```python
from build123d import *

# Parameters (mm, degrees)
BOSS_EXTRUDE1_DEPTH     = 25.5
SKETCH2_R               = 22.5
BOSS_EXTRUDE2_DEPTH     = 100
SKETCH3_W               = 30
SKETCH3_H               = 32
BOSS_EXTRUDE3_DEPTH     = 164.7
SKETCH4_W               = 19
SKETCH4_H               = 20
BOSS_EXTRUDE4_DEPTH     = 20
SKETCH5_R               = 4.05
CUT_EXTRUDE1_DEPTH      = 202.549720913
SKETCH6_R               = 10
BOSS_EXTRUDE5_DEPTH     = 25
SKETCH7_W               = 33
SKETCH7_H               = 35
BOSS_EXTRUDE6_DEPTH     = 13
CUT_EXTRUDE2_DEPTH      = 225.141785484
CUT_EXTRUDE2_DEPTH_BACK = 225.141785484
SKETCH8_R               = 4.05
FILLET1_R               = 2
CUT_EXTRUDE3_START      = -100
SKETCH9_R               = 10
CUT_EXTRUDE3_DEPTH      = 100


with BuildPart() as part:
    # Sketch1 → Boss-Extrude1 (new body)
    with BuildSketch(Plane.XY):
        with BuildLine():
            Line((-22, -4.716990566), (-22, -58.5))
            Line((-22, -58.5), (22, -58.5))
            Line((22, -58.5), (22, -4.716990566))
            ThreePointArc((22, -4.716990566), (0, 22.5), (-22, -4.716990566))
        make_face()
    extrude(amount=BOSS_EXTRUDE1_DEPTH)

    # Sketch2 → Boss-Extrude2 (add)
    with BuildSketch(Plane.XY.offset(25.5)):
        with Locations(Location((0, 0, 0), (0, 0, 192.101492032))):
            Circle(SKETCH2_R)
    extrude(amount=BOSS_EXTRUDE2_DEPTH)

    # Sketch3 → Boss-Extrude3 (add)
    with BuildSketch(Plane.XY.offset(25.5)):
        with Locations((0, -41)):
            Rectangle(SKETCH3_W, SKETCH3_H)
    extrude(amount=BOSS_EXTRUDE3_DEPTH)

    # Sketch4 → Boss-Extrude4 (add)
    with BuildSketch(Plane(origin=(0, 0, 0), x_dir=(-1, 0, 0), z_dir=(0, 0, -1))):
        with Locations((0, -37.7)):
            Rectangle(SKETCH4_W, SKETCH4_H)
    extrude(amount=BOSS_EXTRUDE4_DEPTH)

    # Sketch5 → Cut-Extrude1 (cut, through all)
    with BuildSketch(Plane(origin=(9.5, 0, 0), x_dir=(0, 0, -1), z_dir=(1, 0, 0))):
        with Locations((11, -37.7)):
            Circle(SKETCH5_R)
    extrude(amount=-CUT_EXTRUDE1_DEPTH, mode=Mode.SUBTRACT)

    # Sketch6 → Boss-Extrude5 (add)
    with BuildSketch(Plane.XY.offset(190.2)):
        with Locations((0, -37.7)):
            Circle(SKETCH6_R)
    extrude(amount=BOSS_EXTRUDE5_DEPTH)

    # Sketch7 → Boss-Extrude6 (add)
    with BuildSketch(Plane.XY.offset(190.2)):
        with Locations((0, -41)):
            Rectangle(SKETCH7_W, SKETCH7_H)
    extrude(amount=-BOSS_EXTRUDE6_DEPTH)

    # Sketch8 → Cut-Extrude2 (cut, two sides: drawn at the far end of the back side and taken through both)
    with BuildSketch(Plane(origin=(0, 0, 0), x_dir=(0, 0, -1), z_dir=(1, 0, 0)).offset(-CUT_EXTRUDE2_DEPTH_BACK)):
        with Locations(Location((-205.2, -37.7, 0), (0, 0, 179.999999993))):
            Circle(SKETCH8_R)
    extrude(amount=CUT_EXTRUDE2_DEPTH + CUT_EXTRUDE2_DEPTH_BACK, mode=Mode.SUBTRACT)

    # Fillet1
    fillet1_edges = [part.edges().sort_by_distance(p)[0] for p in [
        (15, -57, 101.35),
        (-15, -57, 101.35),
        (-15, -25, 101.35),
        (15, -25, 101.35),
    ]]
    fillet(fillet1_edges, radius=FILLET1_R)

    # Sketch9 → Cut-Extrude3 (cut)
    with BuildSketch(Plane.XY.offset(215.2).offset(CUT_EXTRUDE3_START)):
        with Locations((0, -37.7)):
            Circle(SKETCH9_R)
    extrude(amount=CUT_EXTRUDE3_DEPTH, mode=Mode.SUBTRACT)


solid = part.part
```
Geometry check sheet. Reference: the model listing, model coordinates, mm. A direction names the side the tool comes from. Give positions to 0.01 mm unless a question says otherwise; leave off trailing zeros. Write each loop counter-clockwise with the first axis right and the second up, starting at its lowest first coordinate (ties: lowest second). Pieces come first, ordered by that corner, then holes.
1) Gauge pin test, flat ends, axial feed: pin 1 (6 mm diameter, centred on x = 3.5, y = -30.5, fed in from +Z); pin 2 (9.5 mm diameter, centred on x = -1.5, z = -8, fed in from +Y); pin 3 (4 mm diameter, centred on x = 0.5, z = 181, fed in from +Y); pin 4 (6 mm diameter, centred on x = 10.5, y = 12.5, fed in from +Z). Record the tip position at first contact, or that the pin passes through.
2) Material ranges on L1, parallel to Y at x = 0.5, z = 73; L2, parallel to Y at x = 4, z = -11; L3, parallel to X at y = -35, z = 2, recorded low to high.
3) Section check B-B, the plane y = -37.7. Record the boundary of the cut face in (x, z), and give its area (3 significant figures).
4) Section check C-C, the plane x = 0. Record the boundary of the cut face in (y, z).
5) Release check for a two-part mould opening along Z. For faces 1 (the flat face through (0, -49, 190.2)), 2 (the flat face through (0, -25, 100)), 3 (the flat face through (0, -47.7, -10)), 4 (the flat face through (-2, -24, 25.5)) record: pulls with the +Z half, pulls with the -Z half, needs draft (parallel to the pull), parting line crosses it, or undercut.
6) Section check A-A, the plane z = 80.5. Record the boundary of the cut face in (x, y).
7) Access from +Z, -Z, +X, -X, +Y, -Y to the whole of each face (thin tool, end or side, straight path). Record for faces 5 (the flat face through (0, 0, 125.5)), 6 (the flat face through (0, -57, 100)), 7 (the flat face through (22, -32, 13)).
8) Section check D-D, the plane z = 148.5. Record the boundary of the cut face in (x, y), and give its area (3 significant figures).
Computed:
1. pin 1: stops at z = 190.2
1. pin 2: stops at y = -27.7
1. pin 3: stops at y = -23.5
1. pin 4: stops at z = 125.5
2. L1: y = -57 to -25, -22.49 to 22.49
2. L2: y = -47.7 to -41.75, -33.65 to -27.7
2. L3: x = -22 to 22
3. outline: (-22, 0) - (-9.5, 0) - (-9.5, -6.95) - (9.5, -6.95) - (9.5, 0) - (22, 0) - (22, 25.5) - (15, 25.5) - (15, 177.2) - (16.5, 177.2) - (16.5, 190.2) - (10, 190.2) - (10, 115.2) - (-10, 115.2) - (-10, 190.2) - (-16.5, 190.2) - (-16.5, 177.2) - (-15, 177.2) - (-15, 25.5) - (-22, 25.5) - close; (-9.5, -20) - (9.5, -20) - (9.5, -15.05) - (-9.5, -15.05) - close
3. area: 4,830 mm2
4. outline: (-58.5, 0) - (-47.7, 0) - (-47.7, -20) - (-27.7, -20) - (-27.7, 0) - (22.5, 0) - (22.5, 125.5) - (-22.5, 125.5) - (-22.5, 25.5) - (-25, 25.5) - (-25, 177.2) - (-23.5, 177.2) - (-23.5, 190.2) - (-27.7, 190.2) - (-27.7, 115.2) - (-47.7, 115.2) - (-47.7, 190.2) - (-58.5, 190.2) - (-58.5, 177.2) - (-57, 177.2) - (-57, 25.5) - (-58.5, 25.5) - close; hole circle Ø8.1 at (-37.7, -11)
5. face 1: pulls with the +Z half
5. face 2: undercut
5. face 3: needs draft
5. face 4: undercut
6. outline: circle Ø45 at (0, 0); (-15, -55) arc R2 ccw to (-13, -57) - (13, -57) arc R2 ccw to (15, -55) - (15, -27) arc R2 ccw to (13, -25) - (-13, -25) arc R2 ccw to (-15, -27) - close
7. face 5: +Z, +X, -X, +Y
7. face 6: +X, -X, -Y
7. face 7: +Z, -Z, +X, -Y
8. outline: (-15, -55) arc R2 ccw to (-13, -57) - (13, -57) arc R2 ccw to (15, -55) - (15, -27) arc R2 ccw to (13, -25) - (-13, -25) arc R2 ccw to (-15, -27) - close; hole circle Ø20 at (0, -37.7)
8. area: 642 mm2
